Can you work these out from the model? Positions are in its coordinate system, mm. A direction names the side the tool comes from. Round coordinates to 2 decimals unless told otherwise and drop trailing zeros. Order: outer loops, then holes, each group sorted by start corner. A loop starts at its lowest first (then second) coordinate and runs counter-clockwise, first axis right, second up. Notation, with made-up numbers: M -13.75,20.25 L 33.25,20.25 A22 ccw 33.25,34.25 Z; hole C -4,71 d11. An arc over 180 degrees is marked long. Answer as a JSON object with one key per item and string values. Group by question number.
```python
from build123d import *

# Parameters (mm, degrees)
CROQUIS1_R              = 4.5
SALIENTE_EXTRUIR1_DEPTH = 25
CROQUIS2_W              = 5
CROQUIS2_H              = 17
SALIENTE_EXTRUIR2_DEPTH = 9
CROQUIS3_R              = 11
CROQUIS3_R_2            = 8
CORTAR_EXTRUIR1_DEPTH   = 9
CROQUIS4_R              = 4.5
SALIENTE_EXTRUIR4_DEPTH = 2
CROQUIS6_W              = 2.5
CROQUIS6_H              = 4
CORTAR_EXTRUIR2_DEPTH   = 5
CROQUIS8_R              = 4.5
SALIENTE_EXTRUIR5_DEPTH = 13
CROQUIS9_R              = 11
SALIENTE_EXTRUIR6_DEPTH = 14


with BuildPart() as part:
    # Croquis1 → Saliente-Extruir1 (new body)
    with BuildSketch(Plane.XY):
        Circle(CROQUIS1_R)
    extrude(amount=SALIENTE_EXTRUIR1_DEPTH)

    # Croquis2 → Saliente-Extruir2 (add)
    with BuildSketch(Plane.XY.offset(25)):
        Rectangle(CROQUIS2_W, CROQUIS2_H)
    extrude(amount=-SALIENTE_EXTRUIR2_DEPTH)

    # Croquis3 → Cortar-Extruir1 (cut)
    with BuildSketch(Plane.XY.offset(25)):
        Circle(CROQUIS3_R)
        Circle(CROQUIS3_R_2, mode=Mode.SUBTRACT)
    extrude(amount=-CORTAR_EXTRUIR1_DEPTH, mode=Mode.SUBTRACT)

    # Croquis4 → Saliente-Extruir4 (add)
    with BuildSketch(Plane(origin=(0, 0, 0), x_dir=(-1, 0, 0), z_dir=(0, 0, -1))):
        Circle(CROQUIS4_R)
    extrude(amount=SALIENTE_EXTRUIR4_DEPTH)

    # Croquis6 → Cortar-Extruir2 (cut)
    with BuildSketch(Plane.XY.offset(25)):
        Rectangle(CROQUIS6_W, CROQUIS6_H)
    extrude(amount=-CORTAR_EXTRUIR2_DEPTH, mode=Mode.SUBTRACT)

    # Croquis8 → Saliente-Extruir5 (add)
    with BuildSketch(Plane(origin=(0, 0, -2), x_dir=(-1, 0, 0), z_dir=(0, 0, -1))):
        Circle(CROQUIS8_R)
    extrude(amount=SALIENTE_EXTRUIR5_DEPTH)

    # Croquis9 → Saliente-Extruir6 (add)
    with BuildSketch(Plane(origin=(0, 0, -15), x_dir=(-1, 0, 0), z_dir=(0, 0, -1))):
        Circle(CROQUIS9_R)
    extrude(amount=SALIENTE_EXTRUIR6_DEPTH)


solid = part.part
```
1) If we section it at B-B on y = -5: Write out the boundary of the cut face in (x, z).
2) I need wall thicknesses on line 1 along Z through (x, y) = (-1.5, -6); line 2 along Z through (x, y) = (6.5, 3.75); line 3 along Y through (x, z) = (-0.25, -17). Which ranges of each line are inside material? Lowest first, please.
3) If we section it at D-D on x = 7.5: Write out the boundary of the cut face in (y, z), plus the area to 3 significant figures.
4) We'd pull the mould along Y, two halves only. Please class faces 1 (the face through (0, 2, 23)), 2 (the face through (0, -8, 21)), 3 (the face through (-2, 0, 25)): +Y half, -Y half, draft (parallel to the pull), parting line (faces both ways), or undercut.
5) If we section it at A-A on x = 0: Write out the boundary of the cut face in (y, z), plus the area to 3 significant figures.
6) If we section it at C-C on y = 0: Write out the boundary of the cut face in (x, z), plus the area to 4 significant figures.
7) For pin 1 (2 mm diameter, centred on y = -0.5, z = 23, fed in from +X); pin 2 (1 mm diameter, centred on x = 3.5, y = -5.5, fed in from +Z); pin 3 (1 mm diameter, centred on x = 1, z = 3.5, fed in from +Y), each with a flat end and sliding along its axis, tell me the tip position at first contact or that it passes through.
8) Which directions (+Z, -Z, +X, -X, +Y, -Y) give clear straight access to the entire face, cutting with the end or side of a thin tool? Please do faces 4 (the face through (0, -5, -15)), 5 (the face through (2.5, -6, 21)), 6 (the face through (0, 0, 20)), 7 (the face through (-2.5, 6, 21)).
Findings:
{
 "1": {"outline": "M -9.8,-29 L 9.8,-29 L 9.8,-15 L -9.8,-15 Z; M -2.5,16 L 2.5,16 L 2.5,25 L -2.5,25 Z"},
 "2": {"line 1": "z = -29 to -15, 16 to 25", "line 2": "z = -29 to -15", "line 3": "y = -11 to 11"},
 "3": {"outline": "M -8.05,-29 L 8.05,-29 L 8.05,-15 L -8.05,-15 Z", "area": "225 mm^2"},
 "4": {"face 1": "undercut", "face 2": "-Y half", "face 3": "draft"},
 "5": {"outline": "M -11,-29 L 11,-29 L 11,-15 L 4.5,-15 L 4.5,16 L 8,16 L 8,25 L 2,25 L 2,20 L -2,20 L -2,25 L -8,25 L -8,16 L -4.5,16 L -4.5,-15 L -11,-15 Z", "area": "711 mm^2"},
 "6": {"outline": "M -11,-29 L 11,-29 L 11,-15 L 4.5,-15 L 4.5,25 L 1.25,25 L 1.25,20 L -1.25,20 L -1.25,25 L -4.5,25 L -4.5,-15 L -11,-15 Z", "area": "655.5 mm^2"},
 "7": {"pin 1": "stops at x = 4.5", "pin 2": "stops at z = -15", "pin 3": "stops at y = 4.47"},
 "8": {"face 4": "none", "face 5": "+Z, +X, -Y", "face 6": "+Z", "face 7": "+Z, -X, +Y"}
}
